For this review, use the dimensioned drawing (mm, ordinates from the lowest corner) and the shaded views. A direction names the side the tool comes from. Coordinates: 2 decimals unless noted, no trailing zeros. Loops run counter-clockwise (first coordinate to the right, second up) from the corner with the lowest first, then second, coordinate; pieces in that order, holes last. Notation, with made-up numbers: M 57.5,24 L 69.5,24 A12 ccw 69.5,36 Z; hole C 57.5,-32 d2. An arc over 180 degrees is marked long. One line per item, written item: value.
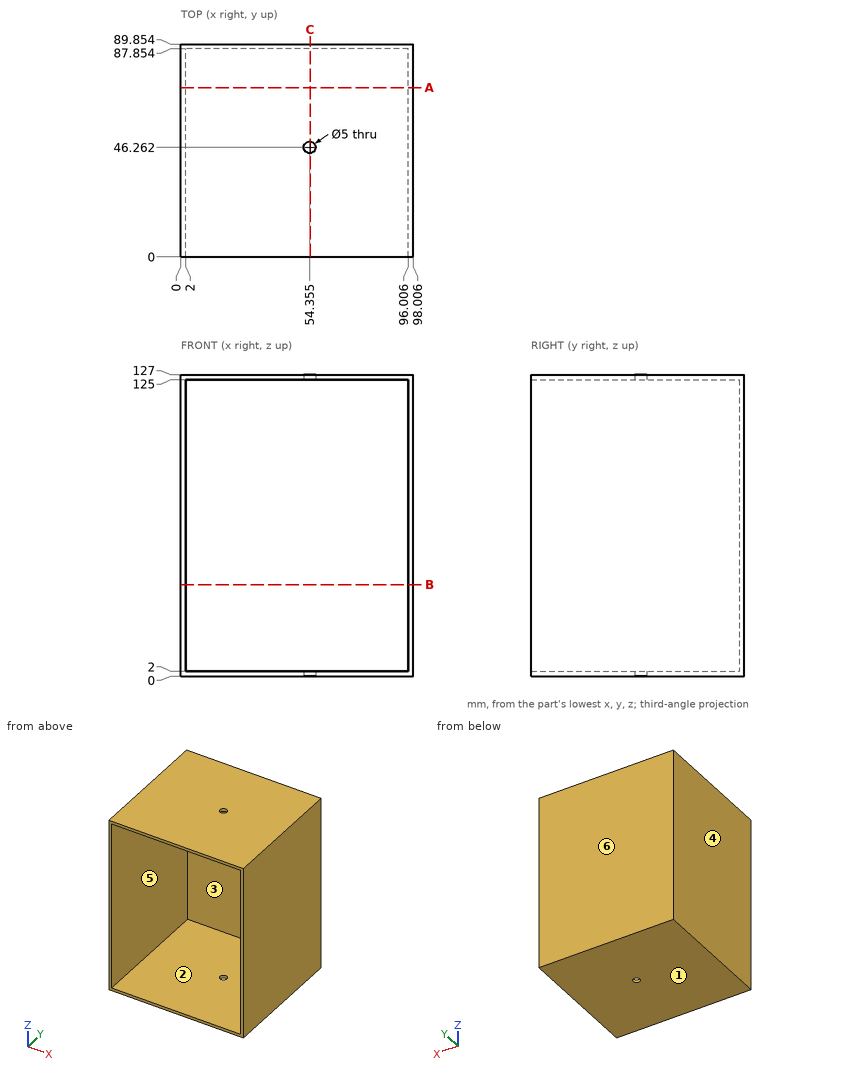
(1) Insertion check: pin 1 (3 mm diameter, centred on x = 54.36, y = 46.26, fed in from +Z). The pin has a flat end and moves straight along its axis. Give the tip position at first contact, or say it passes through.
Reply:
pin 1: passes through
(2) We need section C-C on x = 54.5. State the section outline as (y, z) points (1 decimal).
Reply:
outline: M 0,0 L 43.8,0 L 43.8,2 L 0,2 Z; M 0,125 L 43.8,125 L 43.8,127 L 0,127 Z; M 48.8,0 L 89.9,0 L 89.9,127 L 48.8,127 L 48.8,125 L 87.9,125 L 87.9,2 L 48.8,2 Z
(3) We need section A-A on y = 71.5. State the section outline as (x, z) points.
Reply:
outline: M 0,0 L 98.01,0 L 98.01,127 L 0,127 Z; hole M 2,2 L 96.01,2 L 96.01,125 L 2,125 Z
(4) Mouldability with a two-part tool opening along Z and no side actions: class the marked faces 1, 2, 3 and 4 as released by +Z, released by -Z, zero draft, split by the parting line, or undercut.
Reply:
face 1: released by -Z
face 2: undercut
face 3: undercut
face 4: zero draft
(5) To check wall thickness, follow line 1 along X through (y, z) = (77.5, 73); line 2 along Z through (x, y) = (59.5, 70); line 3 along Y through (x, z) = (58, 104) (1 decimal). State the ranges of each line that lie inside material, in increasing order. Write a range as [from, to].
Reply:
line 1: x = [0, 2], [96.01, 98.01]
line 2: z = [0, 2], [125, 127]
line 3: y = [87.9, 89.9]
(6) Tool access review of the marked faces 5 and 6: name each direction out of +Z, -Z, +X, -X, +Y, -Y from which nothing blocks a thin tool from reaching the whole face with its end or side.
Reply:
face 5: -Y
face 6: +Z, -Z, +X, -X, +Y
(7) We need section B-B on z = 38.5. State the section outline as (x, y) points (1 decimal).
Reply:
outline: M 0,0 L 2,0 L 2,87.9 L 96,87.9 L 96,0 L 98,0 L 98,89.9 L 0,89.9 Z
